Design review of the part built by this model. Coordinates are the model's own, in mm. Face numbers are marked on the shaded views. Coordinates: 2 decimals unless noted, no trailing zeros. Write each loop counter-clockwise with the first axis right and the second up, starting at its lowest first coordinate (ties: lowest second). Pieces come first, ordered by that corner, then holes. Notation, with made-up numbers: M -8,-9.5 L -2,-9.5 A17 ccw -2,18.5 Z; hole C 74,83.25 d3. An arc over 180 degrees is marked long. One line per question, with ' | ' between items.
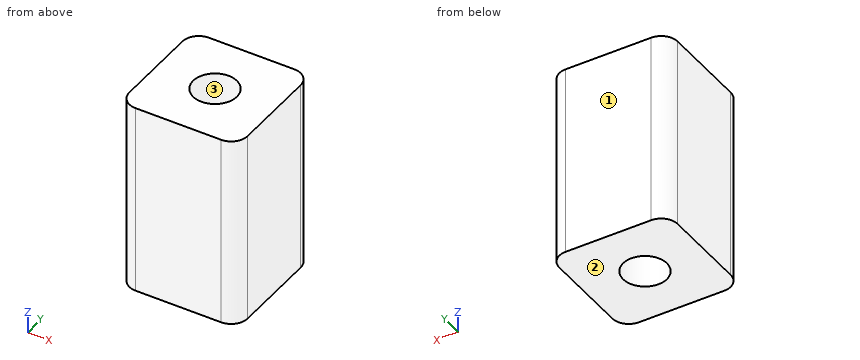
from build123d import *

# Parameters (mm, degrees)
SKETCH_W    = 8.255
SKETCH_H    = 8.255
PAD_DEPTH   = 13.4874
SKETCH001_R = 1.524
HOLE_DEPTH  = 24.9936
FILLET_R    = 1.143


with BuildPart() as part:
    # Sketch → Pad (new body)
    with BuildSketch(Plane.XY):
        Rectangle(SKETCH_W, SKETCH_H)
    extrude(amount=PAD_DEPTH)

    # Sketch001 (on Face6 of Pad) → Hole (cut)
    with BuildSketch(Plane.XY.offset(13.4874)):
        Circle(SKETCH001_R)
    extrude(amount=-HOLE_DEPTH, mode=Mode.SUBTRACT)

    # Fillet
    fillet_edges = [part.edges().sort_by_distance(p)[0] for p in [
        (-4.1275, 4.1275, 6.7437),
        (-4.1275, -4.1275, 6.7437),
        (4.1275, -4.1275, 6.7437),
        (4.1275, 4.1275, 6.7437),
    ]]
    fillet(fillet_edges, radius=FILLET_R)


solid = part.part
1. Draft analysis for pull direction Y (two halves, no side actions). For the marked faces 1, 2 and 3, state which applies: pulls with the +Y half, pulls with the -Y half, needs draft (parallel to the pull), parting line crosses it, or undercut.
Answer sheet:
face 1: pulls with the +Y half | face 2: needs draft | face 3: undercut
2. Take a section at C-C (z = 6.25). Write out the cut boundary in (x, y), then the cut area to 3 significant figures.
Answer sheet:
outline: M -4.13,-2.98 A1.14 ccw -2.98,-4.13 L 2.98,-4.13 A1.14 ccw 4.13,-2.98 L 4.13,2.98 A1.14 ccw 2.98,4.13 L -2.98,4.13 A1.14 ccw -4.13,2.98 Z; hole C 0,0 d3.05 | area: 59.7 mm^2
3. Take a section at A-A (y = 0). Write out the cut boundary in (x, z), then the cut area to 3 significant figures.
Answer sheet:
outline: M -4.13,0 L -1.52,0 L -1.52,13.49 L -4.13,13.49 Z; M 1.52,0 L 4.13,0 L 4.13,13.49 L 1.52,13.49 Z | area: 70.2 mm^2
4. To check wall thickness, follow line 1 along Y through (x, z) = (0, 6); line 2 along X through (y, z) = (0.5, 4.75). State the ranges of each line that lie inside material, in increasing order. Write a range as [from, to].
Answer sheet:
line 1: [-4.13, -1.52], [1.52, 4.13] | line 2: [-4.13, -1.44], [1.44, 4.13]
5. Take a section at D-D (x = 3.75). Write out the cut boundary in (y, z).
Answer sheet:
outline: M -3.83,0 L 3.83,0 L 3.83,13.49 L -3.83,13.49 Z
